The listing builds one solid part. Answer for the finished solid, in the listing's coordinates (mm). Coordinates: 2 decimals unless noted, no trailing zeros. Loops run counter-clockwise (first coordinate to the right, second up) from the corner with the lowest first, then second, coordinate; pieces in that order, holes last. Notation, with made-up numbers: (0, -27.5) - (38, -27.5) arc R27 ccw to (38, -0.5) - close; hole circle Ø3 at (8.5, 0). An arc over 180 degrees is marked (long way). Write each question's results on one line, items separated by ' | '. Start each with the question number.
(1) Consider line 1 (Y direction, x = 61, z = 4.5); line 2 (Y direction, x = 44.5, z = 5.25); line 3 (Y direction, x = 27, z = 1.5). Determine where each line is inside the solid, lowest interval first. Write a range as from..to.
(2) Given pin 1 Ø10 at (x, y) = (58.5, 103) entering from -Z, flat-ended and moving along its own axis, determine where the tip first touches the part or whether it passes through.
(3) Determine the mould class of faces 1 (the cylindrical face through (38.33, 136.52, 3.22)), 2 (the flat face through (38, 165.02, 3)), 3 (the flat face through (0.914, 10, 3)) for opening direction X: released by +X, released by -X, zero draft, split by the parting line, or undercut.
(4) Find section A-A on x = 31. Determine the outline of the cut face in (y, z), then the cut area to 3 significant figures.
(5) Find section B-B on z = 2.75. State how many separate pieces and enclosed holes the cut face has, then the cut area to 3 significant figures.
from build123d import *

# Parameters (mm, degrees)
F0_W      = 76.2
F0_H      = 304.8
F1_DEPTH  = 6.35
F2_R      = 3.175
F3_DEPTH  = 6.35
F4_R      = 14.2875
F5_DEPTH  = 6.35
F6_R      = 14.2875
F7_DEPTH  = 6.35
F8_R      = 2.413
F10_DEPTH = 6.35
F9_R      = 2.413
F11_DEPTH = 6.35


with BuildPart() as f1:
    # F0 (on Top) → F1 (new body)
    with BuildSketch(Plane.XY):
        with Locations((39.014159, 12.620198)):
            Rectangle(F0_W, F0_H)
    extrude(amount=F1_DEPTH)

    # F2 (on face) → F3 (cut)
    with BuildSketch(Plane.XY.offset(6.35)):
        with Locations((39.014159, 139.620198)):
            Circle(F2_R)
    extrude(amount=-F3_DEPTH, mode=Mode.SUBTRACT)

    # F4 (on face) → F5 (cut)
    with BuildSketch(Plane.XY.offset(6.35)):
        with Locations((39.014159, -114.379802)):
            Circle(F4_R)
    extrude(amount=-F5_DEPTH, mode=Mode.SUBTRACT)

    # F6 (on face) → F7 (cut)
    with BuildSketch(Plane.XY.offset(6.35)):
        with Locations((39.014159, 25.320198)):
            Circle(F6_R)
    extrude(amount=-F7_DEPTH, mode=Mode.SUBTRACT)

    # F8 (on face) → F10 (cut)
    with BuildSketch(Plane.XY.offset(6.35)):
        with Locations((61.239159, 7.590998)):
            Circle(F8_R)
    extrude(amount=-F10_DEPTH, mode=Mode.SUBTRACT)

    # F9 (on face) → F11 (cut)
    with BuildSketch(Plane.XY.offset(6.35)):
        with Locations((16.789159, 43.049398)):
            Circle(F9_R)
    extrude(amount=-F11_DEPTH, mode=Mode.SUBTRACT)


solid = f1.part
Values:
1) line 1: y = -139.78..5.19, 9.99..165.02 | line 2: y = -139.78..-127.57, -101.19..12.13, 38.51..165.02 | line 3: y = -139.78..-122.11, -106.65..17.59, 33.05..165.02
2) pin 1: stops at z = 0
3) face 1: undercut | face 2: zero draft | face 3: released by -X
4) outline: (-139.78, 0) - (-126.21, 0) - (-126.21, 6.35) - (-139.78, 6.35) - close; (-102.55, 0) - (13.49, 0) - (13.49, 6.35) - (-102.55, 6.35) - close; (37.15, 0) - (165.02, 0) - (165.02, 6.35) - (37.15, 6.35) - close | area: 1,640 mm²
5) separate pieces: 1 | enclosed holes: 5 | area: 21,900 mm²
